from build123d import *

# Parameters (mm, degrees)
SKETCH1_W          = 58.648623675
SKETCH1_H          = 10.16
BASE_FLANGE1_DEPTH = 0.7874
SKETCH3_R          = 1.3843
CUT_EXTRUDE1_DEPTH = 60.527360581
CUT_EXTRUDE2_DEPTH = 60.527360581
FILLET1_R          = 2.54


# Sheet-metal steps are written as plain solids
with BuildPart() as part:
    # Sketch1 → Base-Flange1 (new body)
    with BuildSketch(Plane(origin=(0, 0, 0), x_dir=(1, 0, 0), z_dir=(0, 1, 0))):
        with Locations((29.324311838, 5.08)):
            Rectangle(SKETCH1_W, SKETCH1_H)
    extrude(amount=-BASE_FLANGE1_DEPTH)

    # Sketch3 → Cut-Extrude1 (cut, through all)
    with BuildSketch(Plane.XZ.offset(0.7874)):
        with Locations(Location((52.793349192, -5.08, 0), (0, 0, 270))):
            Circle(SKETCH3_R)
        with Locations(Location((6.050755325, -5.08, 0), (0, 0, 270))):
            Circle(SKETCH3_R)
    extrude(amount=-CUT_EXTRUDE1_DEPTH, mode=Mode.SUBTRACT)

    # Sketch4 → Cut-Extrude2 (cut, through all)
    with BuildSketch(Plane.XZ.offset(0.7874)):
        Polygon((54.925303053, -10.16), (58.648623675, -10.16), (58.648623675, 0), (56.758255401, 0), align=None)
        Polygon((2.085849116, -10.16), (0, -10.16), (0, 0), (3.918801464, 0), align=None)
    extrude(amount=-CUT_EXTRUDE2_DEPTH, mode=Mode.SUBTRACT)

    # Fillet1
    fillet1_edges = [part.edges().sort_by_distance(p)[0] for p in [
        (3.918801464, -0.3937, 0),
        (2.085849116, -0.3937, -10.16),
        (54.925303053, -0.3937, -10.16),
        (56.758255401, -0.3937, 0),
    ]]
    fillet(fillet1_edges, radius=FILLET1_R)


solid = part.part
Here's how the part is built. I have some questions about the finished solid (model axes, mm). Coordinates: 2 decimals unless noted, no trailing zeros. Order: outer loops, then holes, each group sorted by start corner. A loop starts at its lowest first (then second) coordinate and runs counter-clockwise, first axis right, second up. Notation, with made-up numbers: (63.25, 47) -> (119.25, 47) arc R20 cw to (119.25, 65) -> close; hole circle Ø6 at (-16, 75.5). An arc over 180 degrees is marked (long way). Answer in a Markdown table with one row per item.
(1) I want a section at D-D on z = -1.5. List the corners of the cut face in (x, y) for me.
Answer key:
| item | result |
|---|---|
| outline | (3.72, -0.79) -> (56.04, -0.79) -> (56.04, 0) -> (3.72, 0) -> close |
(2) Please list where these lines run through material, in increasing order: probe 1 along X at (y, z) = (-0.25, -5.08); probe 2 along X at (y, z) = (-0.7, -6.25); probe 3 along X at (y, z) = (-0.15, -2.75).
Answer key:
| item | result |
|---|---|
| probe 1 | 3 to 4.67, 7.44 to 51.41, 54.18 to 55.84 |
| probe 2 | 2.79 to 5.31, 6.79 to 52.05, 53.53 to 55.63 |
| probe 3 | 3.42 to 56.25 |
(3) I want a section at C-C on x = 52. List the corners of the cut face in (y, z) for me.
Answer key:
| item | result |
|---|---|
| outline | (-0.79, -10.16) -> (0, -10.16) -> (0, -6.21) -> (-0.79, -6.21) -> close; (-0.79, -3.95) -> (0, -3.95) -> (0, 0) -> (-0.79, 0) -> close |
(4) I want a section at A-A on z = -5.75. List the corners of the cut face in (x, y) for me.
Answer key:
| item | result |
|---|---|
| outline | (2.88, -0.79) -> (4.84, -0.79) -> (4.84, 0) -> (2.88, 0) -> close; (7.26, -0.79) -> (51.58, -0.79) -> (51.58, 0) -> (7.26, 0) -> close; (54, -0.79) -> (55.72, -0.79) -> (55.72, 0) -> (54, 0) -> close |
(5) I want a section at B-B on y = -0.35. List the corners of the cut face in (x, z) for me, then the cut area to 3 significant figures.
Answer key:
| item | result |
|---|---|
| outline | (2.63, -7.17) arc R2.54 ccw to (5.13, -10.16) -> (52.8, -10.16) arc R2.54 ccw to (55.3, -8.07) -> (56.22, -2.99) arc R2.54 ccw to (53.72, 0) -> (6.04, 0) arc R2.54 ccw to (3.54, -2.09) -> close; hole circle Ø2.77 at (6.05, -5.08); hole circle Ø2.77 at (52.79, -5.08) |
| area | 519 mm^2 |
(6) Will this pin go through, and if not, where does the flat tip stop? pin 1 Ø3.5 at (x, z) = (52.79, -5.08) entering from -Y.
Answer key:
| item | result |
|---|---|
| pin 1 | y = -0.79 |
(7) Thinking about a two-plate mould opening in X: for faces 1 (the face through (3.156, -0.388, -9.225)), 2 (the face through (51.44, -0.4, -4.78)), 3 (the face through (29, 0, -5)), 4 (the face through (55.767, -0.399, -5.495)), which applies, +X half, -X half, draft (parallel to the pull), parting line (faces both ways), or undercut?
Answer key:
| item | result |
|---|---|
| face 1 | -X half |
| face 2 | undercut |
| face 3 | draft |
| face 4 | +X half |
